Geometry check sheet. Reference: the model listing, model coordinates, mm. A direction names the side the tool comes from. Coordinates: 2 decimals unless noted, no trailing zeros. Order: outer loops, then holes, each group sorted by start corner. A loop starts at its lowest first (then second) coordinate and runs counter-clockwise, first axis right, second up. Notation, with made-up numbers: (49.5, 29.5) -> (65.5, 29.5) arc R27 ccw to (65.5, 61.5) -> close; hole circle Ø2 at (-38.5, 76). An arc over 180 degrees is marked (long way). Answer as CSV lines item,"result". Start each with the question number.
Autodesk Inventor part; units mm, degrees
ref_plane "YZ Plane" through (0, 0, 0) normal (1, 0, 0) x (0, 1, 0)
ref_plane "XZ Plane" through (0, 0, 0) normal (0, 1, 0) x (-1, 0, 0)
ref_plane "XY Plane" through (0, 0, 0) normal (0, 0, 1) x (1, 0, 0)
sketch "Boceto1" plane through (0, 0, 0) normal (0, 1, 0) x (-1, 0, 0)
  circle A0 centre (0, 0) radius 6.05
  dimension "d0" = 12.1
extrude "Extrusión1" add sketch "Boceto1" against normal blind 32.7
sketch "Boceto2" plane through (0, 0, 0) normal (0, 1, 0) x (1, 0, 0)
  circle A0 centre (0, 0) radius 4.35
  dimension "d3" = 8.7
extrude "Extrusión2" add sketch "Boceto2" along normal blind 3.7
thread "Rosca1"
sketch "Boceto3" plane through (0, -32.7, 0) normal (0, -1, 0) x (1, 0, 0)
  circle A0 centre (0, 0) radius 6.9
  dimension "d8" = 13.8
sketch "Boceto4" plane through (0, -32.7, 0) normal (0, -1, 0) x (1, 0, 0)
  circle A0 centre (0, 0) radius 5.95
  dimension "d9" = 11.9
extrude "Extrusión3" cut sketch "Boceto4" against normal blind 28.7
sketch "Boceto5" plane through (0, -32.7, 0) normal (0, -1, 0) x (1, 0, 0)
  point P0 (0, 0)
extrude "Extrusión4" add sketch "Boceto3" along normal blind 7.6
sketch "Boceto6" plane through (0, 3.7, 0) normal (0, 1, 0) x (1, 0, 0)
  circle A0 centre (0, 0) radius 1.45
  dimension "d14" = 2.9
extrude "Extrusión5" cut sketch "Boceto6" against normal blind 20
sketch "Boceto7" plane through (0, -40.3, 0) normal (0, -1, 0) x (1, 0, 0)
  circle A0 centre (0, 0) radius 6.85
  circle A1 centre (0, 0) radius 6.9
  dimension "d17" = 13.7
  dimension "d18" = 13.8
extrude "Extrusión6" cut sketch "Boceto7" against normal blind 20
properties part number "Piston(Deposito_deAceite)" material "Plástico ABS"
Q1. Sectioned sample at B-B, the plane z = 0. Record the cut outline in (x, y), then the cut area to 3 significant figures.
Q2. Sectioned sample at A-A, the plane z = 2. Record the cut outline in (x, y), then the cut area to 3 significant figures.
Q3. Sectioned sample at D-D, the plane x = 2.75. Record the cut outline in (y, z), then the cut area to 3 significant figures.
Q4. Access from +Z, -Z, +X, -X, +Y, -Y to the whole of each face (thin tool, end or side, straight path). Record for faces 4 (the flat face through (2, 3.7, 0)), 5 (the cylindrical face through (-0.943, 1.824, -4.247)), 6 (the flat face through (1.2, -4, -1.2)).
Q5. Sectioned sample at C-C, the plane x = 0. Record the cut outline in (y, z), then the cut area to 3 significant figures.
Q6. Thickness scan on L1, parallel to Z at x = 0, y = 1.5; L2, parallel to Y at x = -2, z = -1. Record the ranges inside material, lowest first.
Q7. Release check for a two-part mould opening along X. For faces 1 (the flat face through (-3, 0, -4)), 2 (the flat face through (0, -32.7, 0)), 3 (the cylindrical face through (-5.05, -36.55, 4.63)) record: released by +X, released by -X, zero draft, split by the parting line, or undercut.
Q8. Go/stop test with flat-tipped pins: pin 1 Ø1.5 at (y, z) = (-4.5, 5.5) entering from +X; pin 2 Ø5 at (y, z) = (-11, 1.5) entering from +X; pin 3 Ø8 at (y, z) = (-34, -5) entering from -X. Record where each tip stops, or that it passes through.
Geometry results:
1,outline,"(-6.85, -40.3) -> (6.85, -40.3) -> (6.85, -32.7) -> (6.05, -32.7) -> (6.05, 0) -> (4.35, 0) -> (4.35, 3.7) -> (1.45, 3.7) -> (1.45, -4) -> (5.95, -4) -> (5.95, -32.7) -> (-5.95, -32.7) -> (-5.95, -4) -> (-1.45, -4) -> (-1.45, 3.7) -> (-4.35, 3.7) -> (-4.35, 0) -> (-6.05, 0) -> (-6.05, -32.7) -> (-6.85, -32.7) -> close"
1,area,"168 mm^2"
2,outline,"(-6.55, -40.3) -> (6.55, -40.3) -> (6.55, -32.7) -> (5.71, -32.7) -> (5.71, 0) -> (3.86, 0) -> (3.86, 3.7) -> (-3.86, 3.7) -> (-3.86, 0) -> (-5.71, 0) -> (-5.71, -32.7) -> (-6.55, -32.7) -> close; hole (-5.6, -32.7) -> (5.6, -32.7) -> (5.6, -4) -> (-5.6, -4) -> close"
2,area,"180 mm^2"
3,outline,"(-40.3, -6.27) -> (-32.7, -6.27) -> (-32.7, -5.39) -> (0, -5.39) -> (0, -3.37) -> (3.7, -3.37) -> (3.7, 3.37) -> (0, 3.37) -> (0, 5.39) -> (-32.7, 5.39) -> (-32.7, 6.27) -> (-40.3, 6.27) -> close; hole (-32.7, -5.28) -> (-4, -5.28) -> (-4, 5.28) -> (-32.7, 5.28) -> close"
3,area,"170 mm^2"
4,face 4,"+Z, -Z, +X, -X, +Y"
4,face 5,"+Y"
4,face 6,"none"
5,outline,"(-40.3, -6.85) -> (-32.7, -6.85) -> (-32.7, -6.05) -> (0, -6.05) -> (0, -4.35) -> (3.7, -4.35) -> (3.7, -1.45) -> (-4, -1.45) -> (-4, -5.95) -> (-32.7, -5.95) -> (-32.7, 5.95) -> (-4, 5.95) -> (-4, 1.45) -> (3.7, 1.45) -> (3.7, 4.35) -> (0, 4.35) -> (0, 6.05) -> (-32.7, 6.05) -> (-32.7, 6.85) -> (-40.3, 6.85) -> close"
5,area,"168 mm^2"
6,L1,"z = -4.35 to -1.45, 1.45 to 4.35"
6,L2,"y = -40.3 to -32.7, -4 to 3.7"
7,face 1,"zero draft"
7,face 2,"undercut"
7,face 3,"split by the parting line"
8,pin 1,"stops at x = 3.75"
8,pin 2,"stops at x = 6.05"
8,pin 3,"stops at x = -6.78"
